Autodesk Inventor part; units mm, degrees
ref_plane "YZ Plane" through (0, 0, 0) normal (1, 0, 0) x (0, 1, 0)
ref_plane "XZ Plane" through (0, 0, 0) normal (0, 1, 0) x (-1, 0, 0)
ref_plane "XY Plane" through (0, 0, 0) normal (0, 0, 1) x (1, 0, 0)
sketch "Sketch1" plane through (0, 0, 0) normal (0, 1, 0) x (-1, 0, 0)
  line L0 (0, 0) -> (-41, 0)
  line L1 (-41, 0) -> (-41, -80)
  line L2 (-41, -80) -> (0, -80)
  line L3 (0, -80) -> (0, 0)
  dimension "d0" = 41
  dimension "d1" = 80
extrude "Extrusion1" add sketch "Sketch1" along normal blind 3
sketch "Sketch2" plane through (0, 3, 0) normal (0, 1, 0) x (1, 0, 0)
  line L0 (0, 0) -> (41, 0)
  line L1 (41, 0) -> (25.5, 0)
  line L2 (25.5, 0) -> (25.5, 3)
  line L3 (25.5, 3) -> (41, 3)
  line L4 (41, 3) -> (41, 0)
  line L5 (0, 0) -> (15.5, 0)
  line L6 (15.5, 0) -> (15.5, 3)
  line L7 (15.5, 3) -> (0, 3)
  line L8 (0, 3) -> (0, 0)
  line L9 (0, 3) -> (3, 3)
  line L10 (3, 3) -> (3, 23)
  line L11 (3, 23) -> (0, 23)
  line L12 (0, 23) -> (0, 3)
  line L13 (41, 80) -> (0, 80)
  line L14 (0, 80) -> (3, 80)
  line L15 (3, 80) -> (3, 60)
  line L16 (3, 60) -> (0, 60)
  line L17 (0, 60) -> (0, 80)
  line L18 (41, 3) -> (38, 3)
  line L19 (38, 3) -> (38, 20)
  line L20 (38, 20) -> (41, 20)
  line L21 (41, 20) -> (41, 3)
  line L22 (41, 0) -> (41, 80)
  line L23 (41, 35) -> (38, 35)
  line L24 (38, 35) -> (38, 55)
  line L25 (38, 55) -> (41, 55)
  line L26 (41, 55) -> (41, 35)
  line L27 (41, 80) -> (38, 80)
  line L28 (38, 80) -> (38, 70)
  line L29 (38, 70) -> (41, 70)
  line L30 (41, 70) -> (41, 80)
  dimension "d4" = 15.5
  dimension "d5" = 3
  dimension "d6" = 3
  dimension "d7" = 10
  dimension "d8" = 3
  dimension "d9" = 20
  dimension "d10" = 3
  dimension "d11" = 20
  dimension "d12" = 3
  dimension "d13" = 17
  dimension "d14" = 3
  dimension "d15" = 20
  dimension "d16" = 15
  dimension "d17" = 3
  dimension "d18" = 15
extrude "Extrusion2" cut sketch "Sketch2" against normal through all
sketch "Sketch3" plane through (0, 3, 0) normal (0, 1, 0) x (1, 0, 0)
  line L0 (0, 51) -> (18.5, 51)
  line L1 (18.5, 51) -> (18.5, 38)
  line L2 (18.5, 38) -> (0, 38)
  line L3 (0, 38) -> (0, 51)
  line L4 (15.5, 0) -> (25.5, 0)
  line L5 (18.5, 38) -> (25, 38)
  line L6 (25, 38) -> (25, 41)
  line L7 (25, 41) -> (18.5, 41)
  line L8 (18.5, 41) -> (18.5, 38)
  line L9 (18.5, 51) -> (25, 51)
  line L10 (25, 51) -> (25, 48)
  line L11 (25, 48) -> (18.5, 48)
  line L12 (18.5, 48) -> (18.5, 51)
  line L13 (18.5, 46) -> (25, 46)
  line L14 (25, 46) -> (25, 43)
  line L15 (25, 43) -> (18.5, 43)
  line L16 (18.5, 43) -> (18.5, 46)
  point P0 (0, 0)
  dimension "d21" = 18.5
  dimension "d22" = 13
  dimension "d23" = 38
  dimension "d24" = 6.5
  dimension "d25" = 3
  dimension "d26" = 6.5
  dimension "d27" = 3
  dimension "d28" = 6.5
  dimension "d29" = 3
  dimension "d30" = 2
extrude "Extrusion3" cut sketch "Sketch3" against normal through all contours L9 L10 L11 L1 | L1 L7 L6 L5 | L13 L14 L15 L1
equation "\"d28\" = d24"
equation "\"d29\" = d27"
properties part number "top_right_v2"
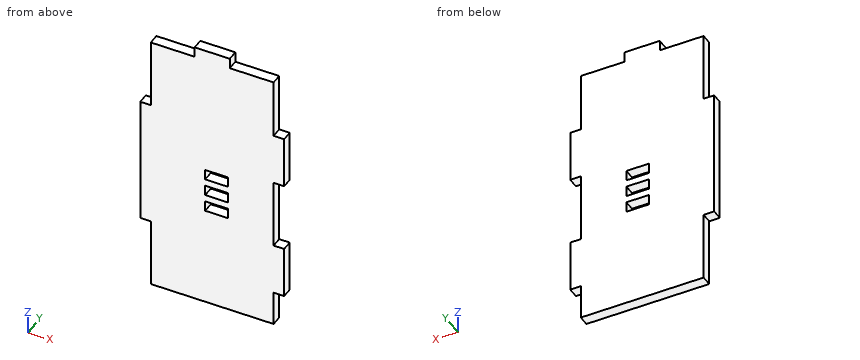
Source: CAD feature listing. Evaluate the final solid. Frame: model axes, mm. Give positions to 0.01 mm unless a question says otherwise; leave off trailing zeros. Loops run counter-clockwise (first coordinate to the right, second up) from the corner with the lowest first, then second, coordinate; pieces in that order, holes last. Notation, with made-up numbers: (60, -38) - (113, -38) arc R33 cw to (113, -4) - close; hole circle Ø2 at (88, 29.5). An arc over 180 degrees is marked (long way). Use CSV: the item, a comma, the result in double quotes.
1) Cut plane A-A (x = 20.5). Output: boundary loops of the cut face in (y, z), and give its area (3 significant figures).
Worked out:
outline,"(0, -80) - (3, -80) - (3, -51) - (0, -51) - close; (0, -48) - (3, -48) - (3, -46) - (0, -46) - close; (0, -43) - (3, -43) - (3, -41) - (0, -41) - close; (0, -38) - (3, -38) - (3, 0) - (0, 0) - close"
area,"213 mm^2"
2) Cut plane B-B (y = 1.35). Count the separate pieces of the cut face and the enclosed holes in it, and give its area (3 significant figures).
Worked out:
separate pieces,"1"
enclosed holes,"3"
area,"2,870 mm^2"
3) Line query: line 1 (Z direction, x = 19, y = 0.95); line 2 (X direction, y = 0.85, z = -50.5); line 3 (Z direction, x = 31, y = 2.5). Output: solid intervals per line, ascending.
Worked out:
line 1,"z = -80 to -51, -48 to -46, -43 to -41, -38 to 0"
line 2,"x = 0 to 18.5, 25 to 38"
line 3,"z = -80 to -3"
4) Pin query (flat end, axial travel): P1, Ø0.9, axis at y = 1.5, z = -76, coming from the +X side; P2, Ø1.5, axis at x = 2, y = 2, coming from the -Z side; P3, Ø1.5, axis at x = 34, y = 1, coming from the +Z side. Return the tip coordinate at first contact, or that it passes through.
Worked out:
P1,"stops at x = 38"
P2,"stops at z = -60"
P3,"stops at z = -3"
5) Cut plane D-D (x = 9.5). Output: boundary loops of the cut face in (y, z).
Worked out:
outline,"(0, -80) - (3, -80) - (3, -3) - (0, -3) - close"
6) Cut plane C-C (z = -10). Output: boundary loops of the cut face in (x, y), and give its area (3 significant figures).
Worked out:
outline,"(3, 0) - (38, 0) - (38, 3) - (3, 3) - close"
area,"105 mm^2"
